The model under review builds one solid part; all positions refer to its coordinate system, in mm. Face numbers are marked on the shaded views. A direction names the side the tool comes from. Round coordinates to 2 decimals unless told otherwise and drop trailing zeros. Loops run counter-clockwise (first coordinate to the right, second up) from the corner with the lowest first, then second, coordinate; pieces in that order, holes last. Notation, with made-up numbers: M -24,29.5 L 8,29.5 A35 cw 8,64.5 Z; hole C 5,4.5 d7. An arc over 180 degrees is marked long. Return JSON: item names as keys, results as strings. Group by question number.
Q1. Draft analysis for pull direction X (two halves, no side actions). For the marked faces 3, 4, 5 and 6, state which applies: pulls with the +X half, pulls with the -X half, needs draft (parallel to the pull), parting line crosses it, or undercut.
Q2. Consider section B-B (z = 0). State the section outline as (x, y) points.
Q3. Clearance check with flat-ended pins moving along their axes: pin 1 Ø4 at (x, y) = (38, -2) entering from +Z; pin 2 Ø2 at (x, y) = (28.5, 15) entering from -Z; pin 3 Ø10 at (y, z) = (14.5, 42) entering from +X. State where each tip first meets the part, or that it passes through.
Q4. Consider section C-C (x = 12.7). State the section outline as (y, z) points.
Q5. Consider section A-A (y = 6.5). State the section outline as (x, z) points.
Q6. To check wall thickness, follow line 1 along X through (y, z) = (-3.55, 0); line 2 along Z through (x, y) = (-12.7, -1.85); line 3 along X through (y, z) = (4.75, 44). State the ranges of each line that lie inside material, in increasing order.
Q7. For the marked faces 1 and 2, list the 3-axis set-ups (+Z, -Z, +X, -X, +Y, -Y) from which the entire face can be reached by the end or side of a thin tool; tool diameter is ignored.
Q8. Consider section D-D (z = 63.5). State the section outline as (x, y) points (1 decimal).
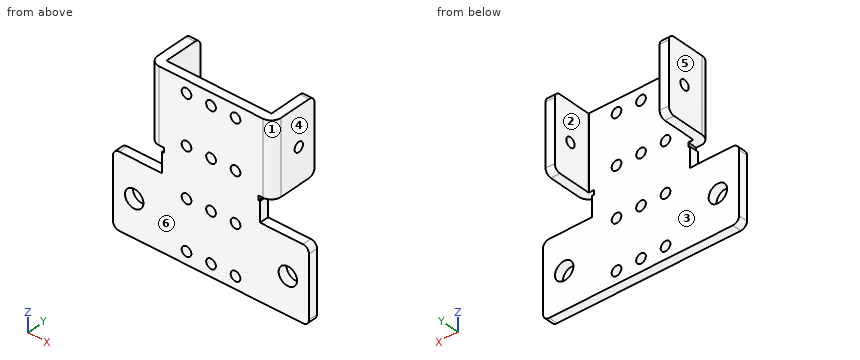
from build123d import *

# Parameters (mm, degrees)
T_LE_DE_BASE_PLI_E1_DEPTH                = 4.76
T_LE_PLI_E_SUR_AR_TE1_STRIP_W            = 19.665
T_LE_PLI_E_SUR_AR_TE1_STRIP_H            = 4.76
T_LE_PLI_E_SUR_AR_TE1_STRIP_CUT_DEPTH    = 38.1
T_LE_PLI_E_SUR_AR_TE1_RELIEF_W           = 22.045
T_LE_PLI_E_SUR_AR_TE1_RELIEF_H           = 2.38
T_LE_PLI_E_SUR_AR_TE1_RELIEF_CUT_DEPTH   = 4.76
T_LE_PLI_E_SUR_AR_TE1_STRIP_2_W          = 19.665
T_LE_PLI_E_SUR_AR_TE1_STRIP_2_H          = 4.76
T_LE_PLI_E_SUR_AR_TE1_STRIP_CUT_2_DEPTH  = 38.1
T_LE_PLI_E_SUR_AR_TE1_RELIEF_2_W         = 22.045
T_LE_PLI_E_SUR_AR_TE1_RELIEF_2_H         = 2.38
T_LE_PLI_E_SUR_AR_TE1_RELIEF_CUT_2_DEPTH = 4.76
T_LE_PLI_E_SUR_AR_TE1_DEPTH              = 38.1
T_LE_PLI_E_SUR_AR_TE1_BEND_DEPTH         = 38.1
ENL_V_MAT_EXTRU_1_REACH                  = 90.709
ESQUISSE12_W                             = 6.54
ESQUISSE12_H                             = 10.32
CONG_1_R                                 = 3.175
ESQUISSE13_R                             = 4.7625
ENL_V_MAT_EXTRU_3_DEPTH                  = 89.709188363
DIAM_TRE_DU_PER_AGE_5_0_5_1_D            = 5
R_P_TITION_LIN_AIRE1_COUNT               = 4
R_P_TITION_LIN_AIRE1_PITCH               = 25.4
DIAM_TRE_DU_PER_AGE_5_0_5_2_D            = 5
DIAM_TRE_DU_PER_AGE_5_0_5_2_DEPTH        = 4.76
DIAM_TRE_DU_PER_AGE_5_0_5_3_D            = 5


# Sheet-metal steps are written as plain solids
with BuildPart() as part:
    # Esquisse1 → Tôle de base pliée1 (new body)
    with BuildSketch(Plane(origin=(0, 0, 0), x_dir=(1, 0, 0), z_dir=(0, 1, 0))):
        Polygon((-31.94, -19.05), (-31.94, -69.85), (31.94, -69.85), (31.94, -19.05), (50.8, -19.05), (50.8, 19.05), (-50.8, 19.05), (-50.8, -19.05), align=None)
    extrude(amount=-T_LE_DE_BASE_PLI_E1_DEPTH)

    # Tôle pliée sur arête1 strip (across the edge) → Tôle pliée sur arête1 strip cut (cut)
    with BuildSketch(Plane(origin=(-31.94, 0, 31.75), x_dir=(1, 0, 0), z_dir=(0, 0, 1))):
        with Locations((-4.76, -2.38)):
            Rectangle(T_LE_PLI_E_SUR_AR_TE1_STRIP_W, T_LE_PLI_E_SUR_AR_TE1_STRIP_H)
    extrude(amount=T_LE_PLI_E_SUR_AR_TE1_STRIP_CUT_DEPTH, mode=Mode.SUBTRACT)

    # Tôle pliée sur arête1 relief (on the sheet) → Tôle pliée sur arête1 relief cut (cut)
    with BuildSketch(Plane(origin=(-26.8675, 0, 31.75), x_dir=(1, 0, 0), z_dir=(0, 1, 0))):
        with Locations((-8.6425, 1.19)):
            Rectangle(T_LE_PLI_E_SUR_AR_TE1_RELIEF_W, T_LE_PLI_E_SUR_AR_TE1_RELIEF_H)
    extrude(amount=-T_LE_PLI_E_SUR_AR_TE1_RELIEF_CUT_DEPTH, mode=Mode.SUBTRACT)

    # Tôle pliée sur arête1 strip 2 (across the edge) → Tôle pliée sur arête1 strip cut 2 (cut)
    with BuildSketch(Plane(origin=(31.94, 0, 69.85), x_dir=(-1, 0, 0), z_dir=(0, 0, -1))):
        with Locations((-4.76, -2.38)):
            Rectangle(T_LE_PLI_E_SUR_AR_TE1_STRIP_2_W, T_LE_PLI_E_SUR_AR_TE1_STRIP_2_H)
    extrude(amount=T_LE_PLI_E_SUR_AR_TE1_STRIP_CUT_2_DEPTH, mode=Mode.SUBTRACT)

    # Tôle pliée sur arête1 relief 2 (on the sheet) → Tôle pliée sur arête1 relief cut 2 (cut)
    with BuildSketch(Plane(origin=(26.8675, 0, 69.85), x_dir=(-1, 0, 0), z_dir=(0, 1, 0))):
        with Locations((-8.6425, -39.29)):
            Rectangle(T_LE_PLI_E_SUR_AR_TE1_RELIEF_2_W, T_LE_PLI_E_SUR_AR_TE1_RELIEF_2_H)
    extrude(amount=-T_LE_PLI_E_SUR_AR_TE1_RELIEF_CUT_2_DEPTH, mode=Mode.SUBTRACT)

    # Tôle pliée sur arête1 section (across the edge) → Tôle pliée sur arête1 (add)
    with BuildSketch(Plane(origin=(-31.94, 0, 31.75), x_dir=(1, 0, 0), z_dir=(0, 0, 1))):
        with BuildLine():
            Line((0, 0.3125), (0, 20.24))
            Line((0, 20.24), (4.76, 20.24))
            Line((4.76, 20.24), (4.76, 0.3125))
            ThreePointArc((4.76, 0.3125), (4.851529131, 0.091529131), (5.0725, 0))
            Line((5.0725, 0), (5.0725, -4.76))
            ThreePointArc((5.0725, -4.76), (1.485700852, -3.274299148), (0, 0.3125))
        make_face()
    extrude(amount=T_LE_PLI_E_SUR_AR_TE1_DEPTH)

    # Tôle pliée sur arête1 section 2 (across the edge) → Tôle pliée sur arête1 bend (add)
    with BuildSketch(Plane(origin=(31.94, 0, 69.85), x_dir=(-1, 0, 0), z_dir=(0, 0, -1))):
        with BuildLine():
            Line((0, 0.3125), (0, 20.24))
            Line((0, 20.24), (4.76, 20.24))
            Line((4.76, 20.24), (4.76, 0.3125))
            ThreePointArc((4.76, 0.3125), (4.851529131, 0.091529131), (5.0725, 0))
            Line((5.0725, 0), (5.0725, -4.76))
            ThreePointArc((5.0725, -4.76), (1.485700852, -3.274299148), (0, 0.3125))
        make_face()
    extrude(amount=T_LE_PLI_E_SUR_AR_TE1_BEND_DEPTH)

    # Esquisse12 → Enlèv. mat.-Extru.1 (cut, up to next)
    with BuildSketch(Plane(origin=(0, 0, 0), x_dir=(1, 0, 0), z_dir=(0, 1, 0)), mode=Mode.PRIVATE) as enl_v_mat_extru_1_sk1:
        with Locations((-28.67, -24.21)):
            Rectangle(ESQUISSE12_W, ESQUISSE12_H)
    enl_v_mat_extru_1_tool1 = extrude(enl_v_mat_extru_1_sk1.sketch, amount=-ENL_V_MAT_EXTRU_1_REACH, mode=Mode.PRIVATE) & part.part
    # Esquisse12 → Enlèv. mat.-Extru.1 (cut, up to next)
    with BuildSketch(Plane(origin=(0, 0, 0), x_dir=(1, 0, 0), z_dir=(0, 1, 0)), mode=Mode.PRIVATE) as enl_v_mat_extru_1_sk2:
        with Locations((28.67, -24.21)):
            Rectangle(ESQUISSE12_W, ESQUISSE12_H)
    enl_v_mat_extru_1_tool2 = extrude(enl_v_mat_extru_1_sk2.sketch, amount=-ENL_V_MAT_EXTRU_1_REACH, mode=Mode.PRIVATE) & part.part
    add(enl_v_mat_extru_1_tool1.solids().sort_by_distance((-28.67, 0, 24.21))[0], mode=Mode.SUBTRACT)
    add(enl_v_mat_extru_1_tool2.solids().sort_by_distance((28.67, 0, 24.21))[0], mode=Mode.SUBTRACT)

    # Congé1
    cong_1_edges = [part.edges().sort_by_distance(p)[0] for p in [
        (-50.8, -2.38, 19.05),
        (-50.8, -2.38, -19.05),
        (50.8, -2.38, -19.05),
        (50.8, -2.38, 19.05),
        (-29.56, 20.24, 31.75),
        (-29.56, 20.24, 69.85),
        (29.56, 20.24, 69.85),
        (29.56, 20.24, 31.75),
    ]]
    fillet(cong_1_edges, radius=CONG_1_R)

    # Esquisse13 → Enlèv. mat.-Extru.3 (cut, through all)
    with BuildSketch(Plane(origin=(0, 0, 0), x_dir=(1, 0, 0), z_dir=(0, 1, 0))):
        with Locations(Location((-39.8145, 0, 0), (0, 0, 270))):
            Circle(ESQUISSE13_R)
        with Locations(Location((39.8145, 0, 0), (0, 0, 90))):
            Circle(ESQUISSE13_R)
    extrude(amount=-ENL_V_MAT_EXTRU_3_DEPTH, mode=Mode.SUBTRACT)

    # Diamètre du perçage Ø5.0 (5)1 (through all)
    with Locations(Plane(origin=(0, 0, 0), x_dir=(1, 0, 0), z_dir=(0, 1, 0))):
        with Locations((-12.7, 12.7), (0, 12.7), (12.7, 12.7)):
            diam_tre_du_per_age_5_0_5_1 = Hole(DIAM_TRE_DU_PER_AGE_5_0_5_1_D / 2)

    # Répétition linéaire1: Diamètre du perçage Ø5.0 (5)1 ×4
    with Locations(*[(0, 0, i * R_P_TITION_LIN_AIRE1_PITCH) for i in range(1, R_P_TITION_LIN_AIRE1_COUNT)]):
        add(diam_tre_du_per_age_5_0_5_1, mode=Mode.SUBTRACT)

    # Diamètre du perçage Ø5.0 (5)2
    with Locations(Plane.ZY.offset(31.94)):
        with Locations((50.06794197, 10.866778695), (38.47565905, -37.875384173)):
            Hole(DIAM_TRE_DU_PER_AGE_5_0_5_2_D / 2, depth=DIAM_TRE_DU_PER_AGE_5_0_5_2_DEPTH)

    # Diamètre du perçage Ø5.0 (5)3 (through all)
    with Locations(Plane(origin=(31.94, 0, 0), x_dir=(0, 0, -1), z_dir=(1, 0, 0))):
        with Locations((-50.06794197, 10.866778695)):
            Hole(DIAM_TRE_DU_PER_AGE_5_0_5_3_D / 2)


solid = part.part
Values:
{
 "1": {"face 3": "undercut", "face 4": "pulls with the +X half", "face 5": "pulls with the -X half", "face 6": "needs draft"},
 "2": {"outline": "M -50.8,-4.76 L -44.58,-4.76 L -44.58,0 L -50.8,0 Z; M -35.05,-4.76 L 35.05,-4.76 L 35.05,0 L -35.05,0 Z; M 44.58,-4.76 L 50.8,-4.76 L 50.8,0 L 44.58,0 Z"},
 "3": {"pin 1": "stops at z = 19.05", "pin 2": "stops at z = 31.75", "pin 3": "stops at x = 31.94"},
 "4": {"outline": "M -4.76,-19.05 L 0,-19.05 L 0,-15.2 L -4.76,-15.2 Z; M -4.76,-10.2 L 0,-10.2 L 0,10.2 L -4.76,10.2 Z; M -4.76,15.2 L 0,15.2 L 0,35.6 L -4.76,35.6 Z; M -4.76,40.6 L 0,40.6 L 0,61 L -4.76,61 Z; M -4.76,66 L 0,66 L 0,69.85 L -4.76,69.85 Z"},
 "5": {"outline": "M -31.94,31.75 L -27.18,31.75 L -27.18,69.85 L -31.94,69.85 Z; M 27.18,31.75 L 31.94,31.75 L 31.94,69.85 L 27.18,69.85 Z"},
 "6": {"line 1": "x = -50.8 to -44.58, -35.05 to 35.05, 44.58 to 50.8", "line 2": "z = -19.05 to -15.2, -10.2 to 10.2, 15.2 to 35.6, 40.6 to 61, 66 to 69.85", "line 3": "x = -31.94 to -27.18, 27.18 to 31.94"},
 "7": {"face 1": "+Z, +X, -Y", "face 2": "+Z, -Z, +Y"},
 "8": {"outline": "M -31.9,0.3 A5.1 ccw -26.9,-4.8 L -15.2,-4.8 L -15.2,0 L -26.9,0 A0.3 cw -27.2,0.3 L -27.2,20.2 L -31.9,20.2 Z; M -10.2,-4.8 L -2.5,-4.8 L -2.5,0 L -10.2,0 Z; M 2.5,-4.8 L 10.2,-4.8 L 10.2,0 L 2.5,0 Z; M 15.2,-4.8 L 26.9,-4.8 A5.1 ccw 31.9,0.3 L 31.9,20.2 L 27.2,20.2 L 27.2,0.3 A0.3 cw 26.9,0 L 15.2,0 Z"}
}
